```python
from build123d import *

# Parameters (mm, degrees)
ESQUISSE1_W             = 44
ESQUISSE1_H             = 22
BOSS_EXTRU_1_DEPTH      = 9
ESQUISSE2_W             = 9
ESQUISSE2_H             = 4.5
BOSS_EXTRU_2_DEPTH      = 4.5
BOSS_EXTRU_2_DEPTH_BACK = 9
CONG_2_R                = 1


with BuildPart() as part:
    # Esquisse1 → Boss.-Extru.1 (new body)
    with BuildSketch(Plane.XY):
        with Locations((22, -11)):
            Rectangle(ESQUISSE1_W, ESQUISSE1_H)
    extrude(amount=BOSS_EXTRU_1_DEPTH)

    # Esquisse2 → Boss.-Extru.2 (add, two sides)
    with BuildSketch(Plane.ZY) as boss_extru_2_sk:
        with Locations((4.5, -2.25)):
            Rectangle(ESQUISSE2_W, ESQUISSE2_H)
    extrude(amount=BOSS_EXTRU_2_DEPTH)
    extrude(boss_extru_2_sk.sketch, amount=-BOSS_EXTRU_2_DEPTH_BACK)

    # Congé2
    cong_2_edges = [part.edges().sort_by_distance(p)[0] for p in [
        (44, -11, 9),
        (19.75, 0, 9),
        (0, -13.25, 0),
        (0, -13.25, 9),
        (-2.25, -4.5, 0),
        (-2.25, -4.5, 9),
        (0, -4.5, 4.5),
        (-4.5, -2.25, 9),
        (-4.5, 0, 4.5),
        (-4.5, -2.25, 0),
        (-4.5, -4.5, 4.5),
        (19.75, 0, 0),
        (44, -11, 0),
        (22, -22, 0),
        (22, -22, 9),
        (44, 0, 4.5),
        (44, -22, 4.5),
        (0, -22, 4.5),
    ]]
    fillet(cong_2_edges, radius=CONG_2_R)


solid = part.part
```
Could you check a few things on this model? Use its own coordinates, in mm. A direction names the side the tool comes from. Coordinates: 2 decimals unless noted, no trailing zeros. Loops run counter-clockwise (first coordinate to the right, second up) from the corner with the lowest first, then second, coordinate; pieces in that order, holes last.
1) Imagine slicing it at A-A (y = -12). List the corners of the cut face in (x, z) for me.
Reported:
outline: (0, 1) arc R1 ccw to (1, 0) - (43, 0) arc R1 ccw to (44, 1) - (44, 8) arc R1 ccw to (43, 9) - (1, 9) arc R1 ccw to (0, 8) - close
2) Please list where these lines run through material, in increasing order: line 1 along X through (y, z) = (-13.5, 8); line 2 along X through (y, z) = (-8.5, 8.75); line 3 along Y through (x, z) = (19.5, 0.5).
Reported:
line 1: x = 0 to 44
line 2: x = 0.34 to 43.66
line 3: y = -21.87 to -0.13
3) Which directions (+Z, -Z, +X, -X, +Y, -Y) give clear straight access to the entire face, cutting with the end or side of a thin tool? Please do faces 1 (the face through (0.301, -13.142, 0.285)), 2 (the face through (-4.5, -2, 4)), 3 (the face through (-2, -4.5, 4)), 4 (the face through (-4.199, -0.285, 4.549)), 5 (the face through (0.301, -13.142, 8.715)).
Reported:
face 1: -Z, -X, -Y
face 2: +Z, -Z, -X, +Y, -Y
face 3: +Z, -Z, -X, -Y
face 4: +Z, -Z, -X, +Y
face 5: +Z, -X, -Y
4) Imagine slicing it at B-B (z = 2). List the corners of the cut face in (x, y) for me.
Reported:
outline: (-4.5, -3.5) arc R1 ccw to (-3.5, -4.5) - (-1, -4.5) arc R1 cw to (0, -5.5) - (0, -21) arc R1 ccw to (1, -22) - (43, -22) arc R1 ccw to (44, -21) - (44, -1) arc R1 ccw to (43, 0) - (-3.5, 0) arc R1 ccw to (-4.5, -1) - close
5) Will these pins go through, and if not, where does the flat tip stop? pin 1 Ø1.2 at (x, z) = (-2.5, 5.5) entering from -Y; pin 2 Ø3.5 at (y, z) = (-14.5, 4) entering from -X.
Reported:
pin 1: stops at y = -4.5
pin 2: stops at x = 0
